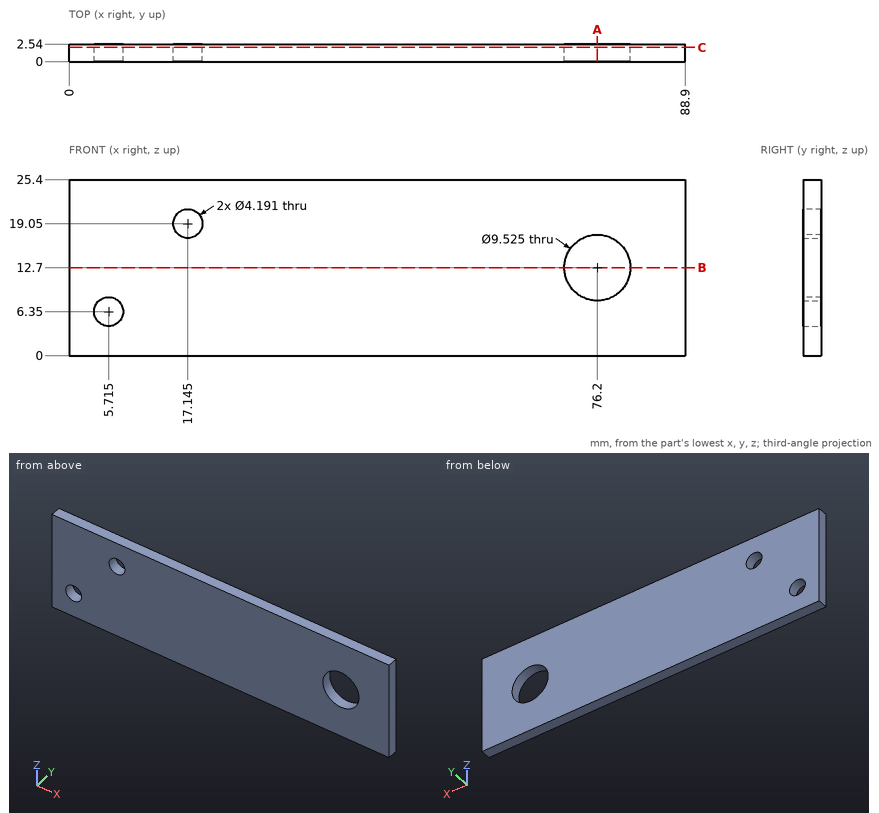
Geometry: see drawing. Coordinates: mm, zero at the bounding-box minimum. Round coordinates to 2 decimals unless told otherwise and drop trailing zeros. Order: outer loops, then holes, each group sorted by start corner. A loop starts at its lowest first (then second) coordinate and runs counter-clockwise, first axis right, second up. Notation, with made-up numbers: (16, 49) - (50, 49) arc R36 ccw to (50, 86) - close; hole circle Ø10 at (6.25, -36). An arc over 180 degrees is marked (long way). Use a Markdown table: item, result. Add a question column.
1. Section query C-C (y = 2.05). Give the number of separate pieces and of enclosed holes in the cut face, then the cut area to 3 significant figures.
2. Section query B-B (z = 12.7). Return the cut outline in (x, y).
3. Line query: probe 1 along X at (y, z) = (0.5, 19.05); probe 2 along X at (y, z) = (0.65, 12.7); probe 3 along Z at (x, y) = (76.2, 2). Output: solid intervals per line, ascending.
4. First-contact query: pin 1 (3.5 mm diameter, centred on x = 5.715, z = 6.35, fed in from +Y); pin 2 (1.5 mm diameter, centred on y = 2, z = 14, fed in from -X). Flat tips, straight axial feed; report the tip coordinate or a pass-through.
5. Section query A-A (x = 76.2). Return the cut outline in (y, z).
Derived:
| question | item | result |
|---|---|---|
| 1 | separate pieces | 1 |
| 1 | enclosed holes | 3 |
| 1 | area | 2,160 mm2 |
| 2 | outline | (0, 0) - (71.44, 0) - (71.44, 2.54) - (0, 2.54) - close; (80.96, 0) - (88.9, 0) - (88.9, 2.54) - (80.96, 2.54) - close |
| 3 | probe 1 | 0 to 15.05, 19.24 to 88.9 |
| 3 | probe 2 | 0 to 71.44, 80.96 to 88.9 |
| 3 | probe 3 | 0 to 7.94, 17.46 to 25.4 |
| 4 | pin 1 | through |
| 4 | pin 2 | x = 0 |
| 5 | outline | (0, 0) - (2.54, 0) - (2.54, 7.94) - (0, 7.94) - close; (0, 17.46) - (2.54, 17.46) - (2.54, 25.4) - (0, 25.4) - close |
